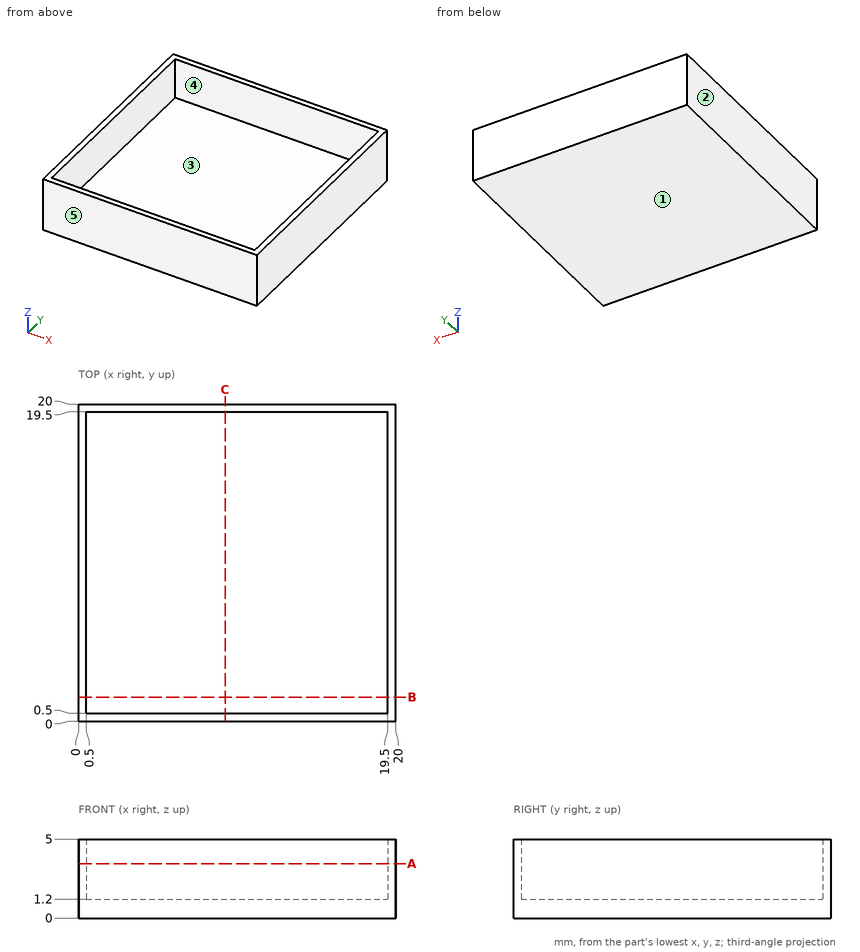
Geometry: see drawing. Coordinates: mm, zero at the bounding-box minimum. A direction names the side the tool comes from. Round coordinates to 2 decimals unless told otherwise and drop trailing zeros. Write each loop counter-clockwise with the first axis right and the second up, starting at its lowest first coordinate (ties: lowest second). Pieces come first, ordered by that corner, then holes. Notation, with made-up numbers: M 10,56 L 28,56 A8 ccw 28,68 Z; hole C 47.25,13.25 d2. An arc over 180 degrees is marked long. Answer in a Markdown table with one row per item. Add a question column.
(1) Draft query along X for the marked faces 1, 2 and 3. Return one class per face: pulls with the +X half, pulls with the -X half, needs draft (parallel to the pull), parting line crosses it, or undercut.
(2) Ray query, L1, parallel to X at y = 9, z = 3.3; L2, parallel to Z at x = 3, y = 14.25. Return the intervals inside material, ascending.
(3) Cut plane B-B, the plane y = 1.5. Return the cut outline in (x, z), then the cut area to 3 significant figures.
(4) Cut plane A-A, the plane z = 3.45. Return the cut outline in (x, y), then the cut area to 3 significant figures.
(5) Contact query for flat-ended pins moving along their axis: pin 1 (1.5 mm diameter, centred on x = 7.5, z = 1.5, fed in from -Y); pin 2 (9.5 mm diameter, centred on x = 14, y = 7.5, fed in from +Z). Output: stop coordinate, or through.
(6) Reachability of the marked faces 4 and 5 from +Z, -Z, +X, -X, +Y, -Y: full face, straight path, thin tool, end or side. Return the list, or none.
Established:
| question | item | result |
|---|---|---|
| 1 | face 1 | needs draft |
| 1 | face 2 | pulls with the -X half |
| 1 | face 3 | undercut |
| 2 | L1 | 0 to 0.5, 19.5 to 20 |
| 2 | L2 | 0 to 1.2 |
| 3 | outline | M 0,0 L 20,0 L 20,5 L 19.5,5 L 19.5,1.2 L 0.5,1.2 L 0.5,5 L 0,5 Z |
| 3 | area | 27.8 mm² |
| 4 | outline | M 0,0 L 20,0 L 20,20 L 0,20 Z; hole M 0.5,0.5 L 19.5,0.5 L 19.5,19.5 L 0.5,19.5 Z |
| 4 | area | 39.0 mm² |
| 5 | pin 1 | y = 0 |
| 5 | pin 2 | z = 1.2 |
| 6 | face 4 | +Z |
| 6 | face 5 | +Z, -Z, +X, -X, -Y |
